Here's how the part is built. I have some questions about the finished solid (model axes, mm). A direction names the side the tool comes from. Coordinates: 2 decimals unless noted, no trailing zeros. Write each loop counter-clockwise with the first axis right and the second up, starting at its lowest first coordinate (ties: lowest second). Pieces come first, ordered by that corner, then holes.
```python
from build123d import *

# Parameters (mm, degrees)
F0_R     = 34.8
F1_DEPTH = 6.35
F2_R     = 24.85
F3_DEPTH = 39
F4_R     = 1
F5_R     = 25.36
F6_DEPTH = 21
F7_R     = 14.86
F8_DEPTH = 10
F10_D    = 16


with BuildPart() as f1:
    # F0 (on Front) → F1 (new body)
    with BuildSketch(Plane.XZ):
        Circle(F0_R)
    extrude(amount=F1_DEPTH)

    # F2 (on face) → F3 (join)
    with BuildSketch(Plane.XZ.offset(6.35)):
        Circle(F2_R)
    extrude(amount=F3_DEPTH)

    # F4
    f4_edges = [f1.edges().sort_by_distance(p)[0] for p in [
        (-24.85, -45.35, 0),
    ]]
    fillet(f4_edges, radius=F4_R)

    # F5 (on face) → F6 (join)
    with BuildSketch(Plane(origin=(0, 0, 0), x_dir=(-1, 0, 0), z_dir=(0, 1, 0))):
        Circle(F5_R)
    extrude(amount=F6_DEPTH)

    # F7 (on face) → F8 (join)
    with BuildSketch(Plane(origin=(0, 21, 0), x_dir=(-1, 0, 0), z_dir=(0, 1, 0))):
        Circle(F7_R)
    extrude(amount=F8_DEPTH)

    # F10 (through all)
    with Locations(Plane.XZ.offset(45.35)):
        with Locations((0, 0)):
            Hole(F10_D / 2)


solid = f1.part
```
1) I need wall thicknesses on probe 1 along Z at (x, y) = (0, 9); probe 2 along Z at (x, y) = (0, -3); probe 3 along Y at (x, z) = (26.5, 2). Which ranges of each line are inside material? Lowest first, please.
Values follow:
probe 1: z = -25.36 to -8, 8 to 25.36
probe 2: z = -34.8 to -8, 8 to 34.8
probe 3: y = -6.35 to 0
2) Imagine slicing it at D-D on y = 5.5. Please give me the cut outline in (x, z).
Values follow:
outline: circle Ø50.72 at (0, 0); hole circle Ø16 at (0, 0)
3) Imagine slicing it at C-C on y = -3. Please give me the cut outline in (x, z), then the cut area to 3 significant figures.
Values follow:
outline: circle Ø69.6 at (0, 0); hole circle Ø16 at (0, 0)
area: 3,600 mm2
4) We'd pull the mould along Z, two halves only. Please class faces 1 (the face through (1.73, -6.64, -7.81)), 2 (the face through (10.952, 25.93, 10.043)), 3 (the face through (-11, 21, -11)): pulls with the +Z half, pulls with the -Z half, needs draft (parallel to the pull), parting line crosses it, or undercut.
Values follow:
face 1: undercut
face 2: parting line crosses it
face 3: needs draft
5) Imagine slicing it at B-B on x = 0. Please give me the cut outline in (y, z).
Values follow:
outline: (-45.35, -23.85) arc R1 ccw to (-44.35, -24.85) - (-6.35, -24.85) - (-6.35, -34.8) - (0, -34.8) - (0, -25.36) - (21, -25.36) - (21, -14.86) - (31, -14.86) - (31, -8) - (-45.35, -8) - close; (-45.35, 8) - (31, 8) - (31, 14.86) - (21, 14.86) - (21, 25.36) - (0, 25.36) - (0, 34.8) - (-6.35, 34.8) - (-6.35, 24.85) - (-44.35, 24.85) arc R1 ccw to (-45.35, 23.85) - close
6) Will these pins go through, and if not, where does the flat tip stop? pin 1 (6 mm diameter, centred on x = 20.5, z = -24.5, fed in from -Y); pin 2 (12 mm diameter, centred on x = -21, z = -25, fed in from +Y); pin 3 (4 mm diameter, centred on x = -15.5, z = 20, fed in from +Y); pin 4 (8 mm diameter, centred on x = 4.5, z = -6.5, fed in from +Y).
Values follow:
pin 1: stops at y = -6.35
pin 2: stops at y = 0
pin 3: stops at y = 21
pin 4: stops at y = 31
7) On a 3-axis mill with a long thin cutter (end or side, diameter ignored), from which of +Z, -Z, +X, -X, +Y, -Y can I reach the whole of each face in a straight line? I mean faces 4 (the face through (-8, -6.35, 24)), 5 (the face through (2, 0, -26)), 6 (the face through (10, -45.35, 0)). Say none if no direction works.
Values follow:
face 4: -Y
face 5: +Y
face 6: +Z, -Z, +X, -X, -Y
8) Imagine slicing it at A-A on z = 0. Please give me the cut outline in (x, y), then the cut area to 3 significant figures.
Values follow:
outline: (-34.8, -6.35) - (-24.85, -6.35) - (-24.85, -44.35) arc R1 ccw to (-23.85, -45.35) - (-8, -45.35) - (-8, 31) - (-14.86, 31) - (-14.86, 21) - (-25.36, 21) - (-25.36, 0) - (-34.8, 0) - close; (8, -45.35) - (23.85, -45.35) arc R1 ccw to (24.85, -44.35) - (24.85, -6.35) - (34.8, -6.35) - (34.8, 0) - (25.36, 0) - (25.36, 21) - (14.86, 21) - (14.86, 31) - (8, 31) - close
area: 2,520 mm2
